Source: CAD feature listing. Evaluate the final solid. Frame: model axes, mm. A direction names the side the tool comes from. Give positions to 0.01 mm unless a question says otherwise; leave off trailing zeros. Order: outer loops, then holes, each group sorted by start corner. A loop starts at its lowest first (then second) coordinate and runs counter-clockwise, first axis right, second up. Notation, with made-up numbers: M 28.25,69 L 84.25,69 A11 ccw 84.25,84 Z; hole C 77.25,-26.75 d10. An arc over 180 degrees is marked long. Answer in a Markdown table with one row per item. Add a question column.
(1) Material intervals for line 1 along X through (y, z) = (30.5, 3.85); line 2 along X through (y, z) = (31, 4.35); line 3 along Y through (x, z) = (-68, 3.5), sorted ascending.
(2) Mould query, pull axis X, two halves, no side actions, for faces 1 (the face through (-70.493, 17.366, 3.74)), 2 (the face through (-110, 29, 1)), 3 (the face through (-30.964, 48.45, 1.232)), 4 (the face through (-66.614, 43.018, 3.493)). Classes: pulls with the +X half, pulls with the -X half, needs draft (parallel to the pull), parting line crosses it, or undercut.
(3) Pin query (flat end, axial travel): P1, Ø5.5, axis at x = -66, y = 31.5, coming from the +Z side. Return the tip coordinate at first contact, or that it passes through.
(4) Section query A-A, the plane z = 1.5. Return loops of the section in (x, y).
(5) Section query B-B, the plane x = -30.5. Return loops of the section in (y, z).
(6) Set-up query: faces 5 (the face through (-26, 28, 1)), 6 (the face through (-79.14, 17.17, 3.49)). Return all of +Z, -Z, +X, -X, +Y, -Y with unobstructed straight access to the full face (end or side cutting, diameter ignored); none if empty.
from build123d import *

# Parameters (mm, degrees)
SKETCH1_R           = 9.5
BOSS_EXTRUDE1_DEPTH = 3
CHAMFER1_SIZE       = 0.5
CUT_EXTRUDE1_REACH  = 124.813
SKETCH2_R           = 1.55
SKETCH3_R           = 1.5
BOSS_EXTRUDE2_DEPTH = 2
CHAMFER2_SIZE       = 1
SKETCH4_R           = 11.5
SKETCH4_R_2         = 9.5
BOSS_EXTRUDE3_DEPTH = 2
CHAMFER3_SIZE       = 0.5


with BuildPart() as part:
    # Sketch1 → Boss-Extrude1 (new body)
    with BuildSketch(Plane.XY):
        Polygon((-110, 14.650482688), (-99.930804426, 2.650482688), (-36.069195574, 2.650482688), (-26, 14.650482688), (-26, 42.534332436), (-36.069195574, 54.534332436), (-99.930804426, 54.534332436), (-110, 42.534332436), align=None)
        with Locations((-68, 28.592407562)):
            Circle(SKETCH1_R, mode=Mode.SUBTRACT)
        with Locations((-68, 28.592407562)):
            Circle(SKETCH1_R)
    extrude(amount=BOSS_EXTRUDE1_DEPTH)

    # Chamfer1
    chamfer1_edges = [part.edges().sort_by_distance(p)[0] for p in [
        (-31.034597787, 8.650482688, 3),
        (-26, 28.592407562, 3),
        (-31.034597787, 48.534332436, 3),
        (-68, 54.534332436, 3),
        (-104.965402213, 48.534332436, 3),
        (-110, 28.592407562, 3),
        (-104.965402213, 8.650482688, 3),
        (-68, 2.650482688, 3),
    ]]
    chamfer(chamfer1_edges, length=CHAMFER1_SIZE)

    # Sketch2 → Cut-Extrude1 (cut, up to next)
    with BuildSketch(Plane(origin=(0, 0, 0), x_dir=(-1, 0, 0), z_dir=(0, 0, -1)), mode=Mode.PRIVATE) as cut_extrude1_sk1:
        with Locations((40.392445123, 45.685066176)):
            Circle(SKETCH2_R)
    cut_extrude1_tool1 = extrude(cut_extrude1_sk1.sketch, amount=-CUT_EXTRUDE1_REACH, mode=Mode.PRIVATE) & part.part
    # Sketch2 → Cut-Extrude1 (cut, up to next)
    with BuildSketch(Plane(origin=(0, 0, 0), x_dir=(-1, 0, 0), z_dir=(0, 0, -1)), mode=Mode.PRIVATE) as cut_extrude1_sk2:
        with Locations((95.607554877, 45.685066176)):
            Circle(SKETCH2_R)
    cut_extrude1_tool2 = extrude(cut_extrude1_sk2.sketch, amount=-CUT_EXTRUDE1_REACH, mode=Mode.PRIVATE) & part.part
    # Sketch2 → Cut-Extrude1 (cut, up to next)
    with BuildSketch(Plane(origin=(0, 0, 0), x_dir=(-1, 0, 0), z_dir=(0, 0, -1)), mode=Mode.PRIVATE) as cut_extrude1_sk3:
        with Locations((95.607554877, 11.499748948)):
            Circle(SKETCH2_R)
    cut_extrude1_tool3 = extrude(cut_extrude1_sk3.sketch, amount=-CUT_EXTRUDE1_REACH, mode=Mode.PRIVATE) & part.part
    # Sketch2 → Cut-Extrude1 (cut, up to next)
    with BuildSketch(Plane(origin=(0, 0, 0), x_dir=(-1, 0, 0), z_dir=(0, 0, -1)), mode=Mode.PRIVATE) as cut_extrude1_sk4:
        with Locations((40.392445123, 11.499748948)):
            Circle(SKETCH2_R)
    cut_extrude1_tool4 = extrude(cut_extrude1_sk4.sketch, amount=-CUT_EXTRUDE1_REACH, mode=Mode.PRIVATE) & part.part
    add(cut_extrude1_tool1.solids().sort_by_distance((-40.392445, 45.685066, 0))[0], mode=Mode.SUBTRACT)
    add(cut_extrude1_tool2.solids().sort_by_distance((-95.607555, 45.685066, 0))[0], mode=Mode.SUBTRACT)
    add(cut_extrude1_tool3.solids().sort_by_distance((-95.607555, 11.499749, 0))[0], mode=Mode.SUBTRACT)
    add(cut_extrude1_tool4.solids().sort_by_distance((-40.392445, 11.499749, 0))[0], mode=Mode.SUBTRACT)

    # Sketch3 → Boss-Extrude2 (add)
    with BuildSketch(Plane.XY.offset(3)):
        with Locations((-68, 43.592407562)):
            Circle(SKETCH3_R)
        with Locations((-62.86969785, 42.687796874)):
            Circle(SKETCH3_R)
        with Locations((-58.358185855, 40.083074209)):
            Circle(SKETCH3_R)
        with Locations((-55.009618943, 36.092407562)):
            Circle(SKETCH3_R)
        with Locations((-53.227883705, 31.197130227)):
            Circle(SKETCH3_R)
        with Locations((-53.227883705, 25.987684897)):
            Circle(SKETCH3_R)
        with Locations((-55.009618943, 21.092407562)):
            Circle(SKETCH3_R)
        with Locations((-58.358185855, 17.101740915)):
            Circle(SKETCH3_R)
        with Locations((-62.86969785, 14.49701825)):
            Circle(SKETCH3_R)
        with Locations((-68, 13.592407562)):
            Circle(SKETCH3_R)
        with Locations((-73.13030215, 14.49701825)):
            Circle(SKETCH3_R)
        with Locations((-77.641814145, 17.101740915)):
            Circle(SKETCH3_R)
        with Locations((-80.990381057, 21.092407562)):
            Circle(SKETCH3_R)
        with Locations((-82.772116295, 25.987684897)):
            Circle(SKETCH3_R)
        with Locations((-82.772116295, 31.197130227)):
            Circle(SKETCH3_R)
        with Locations((-80.990381057, 36.092407562)):
            Circle(SKETCH3_R)
        with Locations((-77.641814145, 40.083074209)):
            Circle(SKETCH3_R)
        with Locations((-73.13030215, 42.687796874)):
            Circle(SKETCH3_R)
    extrude(amount=BOSS_EXTRUDE2_DEPTH)

    # Chamfer2
    chamfer2_edges = [part.edges().sort_by_distance(p)[0] for p in [
        (-79.141814145, 17.101740915, 5),
        (-82.490381057, 21.092407562, 5),
        (-84.272116295, 25.987684897, 5),
        (-84.272116295, 31.197130227, 5),
        (-82.490381057, 36.092407562, 5),
        (-79.141814145, 40.083074209, 5),
        (-74.63030215, 14.49701825, 5),
        (-74.63030215, 42.687796874, 5),
        (-69.5, 43.592407562, 5),
        (-64.36969785, 42.687796874, 5),
        (-59.858185855, 40.083074209, 5),
        (-56.509618943, 36.092407562, 5),
        (-54.727883705, 31.197130227, 5),
        (-54.727883705, 25.987684897, 5),
        (-56.509618943, 21.092407562, 5),
        (-59.858185855, 17.101740915, 5),
        (-64.36969785, 14.49701825, 5),
        (-69.5, 13.592407562, 5),
    ]]
    chamfer(chamfer2_edges, length=CHAMFER2_SIZE)

    # Sketch4 → Boss-Extrude3 (add)
    with BuildSketch(Plane.XY.offset(3)):
        with Locations((-68, 28.592407562)):
            Circle(SKETCH4_R)
        with Locations((-68, 28.592407562)):
            Circle(SKETCH4_R_2, mode=Mode.SUBTRACT)
    extrude(amount=BOSS_EXTRUDE3_DEPTH)

    # Chamfer3
    chamfer3_edges = [part.edges().sort_by_distance(p)[0] for p in [
        (-77.5, 28.592407562, 5),
        (-79.5, 28.592407562, 5),
    ]]
    chamfer(chamfer3_edges, length=CHAMFER3_SIZE)


solid = part.part
Values follow:
| question | item | result |
|---|---|---|
| 1 | line 1 | x = -84.1 to -81.44, -79.34 to -77.31, -58.69 to -56.66, -54.56 to -51.9 |
| 1 | line 2 | x = -83.91 to -81.64, -79.25 to -77.19, -58.81 to -56.75, -54.36 to -52.09 |
| 1 | line 3 | y = 12.09 to 15.09, 17.09 to 19.09, 38.09 to 40.09, 42.09 to 45.09 |
| 2 | face 1 | undercut |
| 2 | face 2 | pulls with the -X half |
| 2 | face 3 | pulls with the +X half |
| 2 | face 4 | undercut |
| 3 | P1 | stops at z = 3 |
| 4 | outline | M -110,14.65 L -99.93,2.65 L -36.07,2.65 L -26,14.65 L -26,42.53 L -36.07,54.53 L -99.93,54.53 L -110,42.53 Z; hole C -95.61,11.5 d3.1; hole C -95.61,45.69 d3.1; hole C -40.39,11.5 d3.1; hole C -40.39,45.69 d3.1 |
| 5 | outline | M 9.29,0 L 47.9,0 L 47.9,2.5 L 47.12,3 L 10.07,3 L 9.29,2.5 Z |
| 6 | face 5 | +Z, -Z, +X, +Y, -Y |
| 6 | face 6 | +Z |
